```python
from build123d import *

# Parameters (mm, degrees)
BASPROSKE_W              = 15
BASPROSKE_H              = 12
TOOTHCUT_DEPTH           = 23.649503306
TEETHCUTS_COUNT          = 14
TEETHCUTS_ANGLE          = 334.285714286
BORSKE_R                 = 4
BORE_DEPTH               = 50.0000508
ESBO_O3_R                = 4
ESBO_O3_R_2              = 3
RESSALTO_EXTRUS_O2_DEPTH = 15
ESBO_O4_R                = 14.250212497
CORTE_EXTRUS_O2_DEPTH    = 5
CORTE_EXTRUS_O3_DEPTH    = 20.555988541
ESBO_O7_R                = 6.5
RESSALTO_EXTRUS_O4_DEPTH = 2


with BuildPart() as part:
    # BasProSke → Base-Revolve (revolve)
    with BuildSketch(Plane(origin=(0, 0, 0), x_dir=(1, 0, 0), z_dir=(0, 1, 0)), mode=Mode.PRIVATE) as base_revolve_sk:
        with Locations((7.5, 6)):
            Rectangle(BASPROSKE_W, BASPROSKE_H)
    revolve(base_revolve_sk.sketch.rotate(Axis((-10, 0, 0), (1, 0, 0)), 180), axis=Axis((-10, 0, 0), (1, 0, 0)))

    # TooCutSke → ToothCut (cut, through all)
    with BuildSketch(Plane(origin=(0, 0, 0), x_dir=(0, 0, -1), z_dir=(1, 0, 0))):
        with BuildLine():
            ThreePointArc((0.804845511, 8.586361261), (0, 8.624), (-0.804845511, 8.586361261))
            ThreePointArc((-0.804845511, 8.586361261), (-1.237812142, 10.362618414), (-2.384428228, 11.78663426))
            ThreePointArc((-2.384428228, 11.78663426), (0, 12.0254), (2.384428228, 11.78663426))
            ThreePointArc((2.384428228, 11.78663426), (1.237812142, 10.362618414), (0.804845511, 8.586361261))
        make_face()
    toothcut = extrude(amount=TOOTHCUT_DEPTH, mode=Mode.SUBTRACT)

    # TeethCuts: ToothCut ×14 about axis
    teethcuts_axis = Axis((-10, 0, 0), (1, 0, 0))
    for i in range(1, TEETHCUTS_COUNT):
        add(toothcut.rotate(teethcuts_axis, i * TEETHCUTS_ANGLE / (TEETHCUTS_COUNT - 1)), mode=Mode.SUBTRACT)

    # BorSke → Bore (cut, symmetric)
    with BuildSketch(Plane(origin=(0, 0, 0), x_dir=(0, 0, -1), z_dir=(1, 0, 0))):
        with Locations(Location((0, 0, 0), (0, 0, 180))):
            Circle(BORSKE_R)
    extrude(amount=BORE_DEPTH, both=True, mode=Mode.SUBTRACT)

    # Esboço3 → Ressalto-extrusão2 (add)
    with BuildSketch(Plane(origin=(15, 0, 0), x_dir=(0, 0, -1), z_dir=(1, 0, 0))):
        Circle(ESBO_O3_R)
        Circle(ESBO_O3_R_2, mode=Mode.SUBTRACT)
    extrude(amount=-RESSALTO_EXTRUS_O2_DEPTH)

    # Esboço4 → Corte-extrusão2 (cut)
    with BuildSketch(Plane(origin=(15, 0, 0), x_dir=(0, 0, -1), z_dir=(1, 0, 0))):
        Circle(ESBO_O4_R)
    extrude(amount=-CORTE_EXTRUS_O2_DEPTH, mode=Mode.SUBTRACT)

    # Esboço5 → Corte-extrusão3 (cut, through all)
    with BuildSketch(Plane.ZY):
        Polygon((4.156921938, 2.4), (0, 4.8), (-4.156921938, 2.4), (-4.156921938, -2.4), (0, -4.8), (4.156921938, -2.4), align=None)
    extrude(amount=-CORTE_EXTRUS_O3_DEPTH, mode=Mode.SUBTRACT)

    # Esboço7 → Ressalto-extrusão4 (add)
    with BuildSketch(Plane.ZY):
        with Locations(Location((0, 0, 0), (0, 0, 180))):
            Circle(ESBO_O7_R)
        Polygon((0, 4.8), (-4.156921938, 2.4), (-4.156921938, -2.4), (0, -4.8), (4.156921938, -2.4), (4.156921938, 2.4), align=None, mode=Mode.SUBTRACT)
    extrude(amount=RESSALTO_EXTRUS_O4_DEPTH)


solid = part.part
```
Can you work these out from the model? Positions are in its coordinate system, mm. A direction names the side the tool comes from. Give positions to 0.01 mm unless a question says otherwise; leave off trailing zeros. Loops run counter-clockwise (first coordinate to the right, second up) from the corner with the lowest first, then second, coordinate; pieces in that order, holes last. Notation, with made-up numbers: M -23,-36.5 L 25,-36.5 A18 ccw 25,-3.5 Z; hole C 9.25,57.5 d4. An arc over 180 degrees is marked long. Use one line per item in the form item = value. Start each with the question number.
(1) I want a section at C-C, the plane y = -3.5. Write out the boundary of the cut face in (x, z), and give its area (3 significant figures).
(2) I'm going to push flat-ended pins straight in: P1, Ø1.5, axis at x = 1.5, z = 7, coming from the +Y side; P2, Ø2, axis at x = 8, z = -3.5, coming from the +Y side; P3, Ø2, axis at x = -0.5, y = -6.5, coming from the -Z side. Where does each tip first touch, or does it pass through?
(3) On a 3-axis mill with a long thin cutter (end or side, diameter ignored), from which of +Z, -Z, +X, -X, +Y, -Y can I reach the whole of each face in a straight line? I mean faces 4 (the cylindrical face through (4.93, 10.37, -1.24)), 5 (the cylindrical face through (4.93, -1.097, 10.387)), 6 (the cylindrical face through (4.93, -8.805, 5.619)). Say none if no direction works.
(4) I want a section at B-B, the plane z = -9.25. Write out the boundary of the cut face in (x, y).
(5) Thinking about a two-plate mould opening in Z: for faces 1 (the cylindrical face through (4.93, -3.486, 9.795)), 2 (the cylindrical face through (4.93, 7.775, 3.732)), 3 (the cylindrical face through (4.93, -3.518, -9.834)), which applies, released by +Z, released by -Z, zero draft, split by the parting line, or undercut?
(6) Please list where these lines run through material, in increasing order: line 1 (Y direction, x = 2.5, z = 7.25); line 2 (Z direction, x = 6.25, y = -5.25); line 3 (Y direction, x = 2.25, z = -9.75).
(7) I want a section at A-A, the plane y = 0. Write out the boundary of the cut face in (x, z).
Worked out:
q1.outline = M -2,-5.48 L 0,-5.48 L 0,-9.81 L 10,-9.81 L 10,-2.25 L -2,-2.25 Z; M -2,2.25 L 10,2.25 L 10,9.81 L 0,9.81 L 0,5.48 L -2,5.48 Z
q1.area = 164 mm²
q2.P1 = 9.58
q2.P2 = 11.74
q2.P3 = -7.3
q3.face_4 = +X, -X, +Y
q3.face_5 = +X, -X
q3.face_6 = +X, -X, -Y
q4.outline = M 0,-5.56 L 10,-5.56 L 10,-3.12 L 0,-3.12 Z; M 0,-1.21 L 10,-1.21 L 10,1.21 L 0,1.21 Z; M 0,3.12 L 10,3.12 L 10,5.56 L 0,5.56 Z
q5.face_1 = released by +Z
q5.face_2 = undercut
q5.face_3 = released by -Z
q6.line_1 = -9.56 to -7.27, -4.75 to 4.75, 7.27 to 9.56
q6.line_2 = -10.79 to -8.11, -6.84 to 6.84, 8.11 to 10.79
q6.line_3 = -5.59 to -3.45, -1.2 to 1.2, 3.45 to 5.59
q7.outline = M -2,-6.5 L 0,-6.5 L 0,-12 L 10,-12 L 10,-4.16 L -2,-4.16 Z; M -2,4.16 L 10,4.16 L 10,12 L 0,12 L 0,6.5 L -2,6.5 Z
